Part model, mm, in its own coordinate system. Face numbers are marked on the shaded views. A direction names the side the tool comes from. Give positions to 0.01 mm unless a question says otherwise; leave off trailing zeros. Order: outer loops, then holes, each group sorted by start corner. A loop starts at its lowest first (then second) coordinate and runs counter-clockwise, first axis right, second up. Notation, with made-up numbers: (12.25, 4.25) -> (34.25, 4.25) arc R16 cw to (34.25, 30.25) -> close; hole circle Ø11 at (20, -1.5). An arc over 180 degrees is marked (long way). Write item = value, one per line. Start each with the question number.
Item 1: Band-saw the part on D-D on y = -137.5. Write the cut outline in (x, z), plus the area to 3 significant figures.
Item 2: Pull direction Z, two halves, no side cores. Call the marked faces 3, 4 and 5: +Z half, -Z half, draft (parallel to the pull), parting line (faces both ways), or undercut.
Item 3: Tool access for the marked faces 1 and 2: list every direction of +Z, -Z, +X, -X, +Y, -Y with a clear straight run to the whole face (end or side of a thin tool).
Item 4: Band-saw the part on A-A on y = -17.5. Write the cut outline in (x, z).
Item 5: Band-saw the part on B-B on z = 0. Write the cut outline in (x, y), plus the area to 3 significant figures.
Item 6: Band-saw the part on C-C on y = -70.5. Write the cut outline in (x, z).
Item 7: Flat gauge pins, fed straight in: P1, Ø18.5, axis at y = -13.5, z = -18, coming from the -X side; P2, Ø6, axis at x = 0, y = -126, coming from the -Z side; P3, Ø8, axis at x = 18, y = -43, coming from the +Z side. Where does each tip first touch, or does it go through?
Item 8: Drill centre lines: line 1 along X through (y, z) = (-29.5, 0); line 2 along Y through (x, z) = (0, 10). Where is each one in solid material? Low to high.
```python
from build123d import *

# Parameters (mm, degrees)
STOCKDIAMETER_R        = 22.5
BASESTOCK_DEPTH        = 150
DIAMETERCUT_START      = -25
SKETCH11_OUTSIDE_W     = 79.588
SKETCH11_OUTSIDE_H     = 79.588
SKETCH11_OUTSIDE_R     = 17.5
DIAMETERCUT_DEPTH      = 126
SHAFTHOLE_R            = 6
MOTOR1SHAFTHOLE_DEPTH  = 151
SKETCH10_W             = 4
SKETCH10_H             = 20
SHAFTKEY_DEPTH         = 23.5
SHAFTKEY_DEPTH_BACK    = 23.5
ARMKEY_START           = -150
ARMKEYSKETCH_W         = 60
ARMKEYSKETCH_H         = 20
ARMKEY_DEPTH           = 50
ARM1MOUNTINGHOLE_START = 15
SKETCH13_R             = 5
ARM1MOUNTINGHOLE_DEPTH = 11.683375
FILLET1_R              = 1


with BuildPart() as part:
    # StockDiameter → BaseStock (new body)
    with BuildSketch(Plane(origin=(0, 0, 0), x_dir=(1, 0, 0), z_dir=(0, 1, 0))):
        Circle(STOCKDIAMETER_R)
    extrude(amount=-BASESTOCK_DEPTH)

    # Sketch11 outside → DiameterCut (cut, through all)
    with BuildSketch(Plane(origin=(0, 0, 0), x_dir=(1, 0, 0), z_dir=(0, 1, 0)).offset(DIAMETERCUT_START)):
        Rectangle(SKETCH11_OUTSIDE_W, SKETCH11_OUTSIDE_H)
        Circle(SKETCH11_OUTSIDE_R, mode=Mode.SUBTRACT)
    extrude(amount=-DIAMETERCUT_DEPTH, mode=Mode.SUBTRACT)

    # ShaftHole → Motor1ShaftHole (cut, through all)
    with BuildSketch(Plane(origin=(0, 0, 0), x_dir=(1, 0, 0), z_dir=(0, 1, 0))):
        Circle(SHAFTHOLE_R)
    extrude(amount=-MOTOR1SHAFTHOLE_DEPTH, mode=Mode.SUBTRACT)

    # Sketch10 → ShaftKey (cut, two sides)
    with BuildSketch(Plane.XY) as shaftkey_sk:
        with Locations((0, -10)):
            Rectangle(SKETCH10_W, SKETCH10_H)
    extrude(amount=SHAFTKEY_DEPTH, mode=Mode.SUBTRACT)
    extrude(shaftkey_sk.sketch, amount=-SHAFTKEY_DEPTH_BACK, mode=Mode.SUBTRACT)

    # ArmKeySketch → ArmKey (cut)
    with BuildSketch(Plane(origin=(0, 0, 0), x_dir=(1, 0, 0), z_dir=(0, 1, 0)).offset(ARMKEY_START)):
        with Locations((0, -25)):
            Rectangle(ARMKEYSKETCH_W, ARMKEYSKETCH_H)
    extrude(amount=ARMKEY_DEPTH, mode=Mode.SUBTRACT)

    # Sketch13 → Arm1MountingHole (cut)
    with BuildSketch(Plane.XY.offset(ARM1MOUNTINGHOLE_START)):
        with Locations((0, -126)):
            Circle(SKETCH13_R)
    extrude(amount=-ARM1MOUNTINGHOLE_DEPTH, mode=Mode.SUBTRACT)

    # Fillet1
    fillet1_edges = [part.edges().sort_by_distance(p)[0] for p in [
        (-22.5, -25, 0),
    ]]
    fillet(fillet1_edges, radius=FILLET1_R)


solid = part.part
```
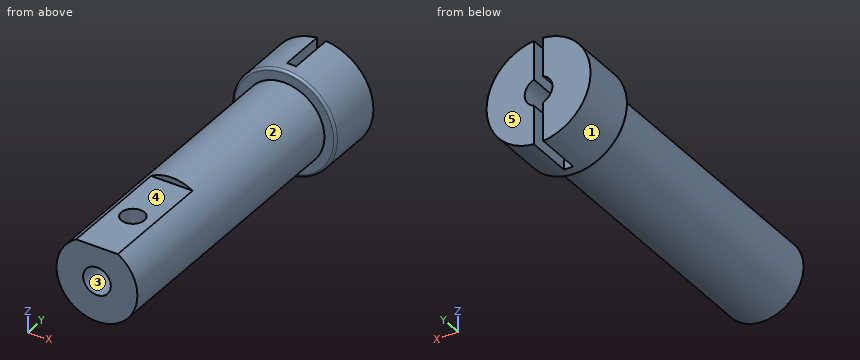
Values found:
q1.outline = (-9.01, 15) arc R17.5 ccw (long way) to (9.01, 15) -> close; hole circle Ø12 at (0, 0)
q1.area = 819 mm^2
q2.face_3 = undercut
q2.face_4 = +Z half
q2.face_5 = draft
q3.face_1 = +Y, -Y
q3.face_2 = -Y
q4.outline = (-2, -22.41) -> (-2, -5.66) arc R6 cw to (-2, 5.66) -> (-2, 22.41) arc R22.5 ccw to start; (2, -22.41) arc R22.5 ccw to (2, 22.41) -> (2, 5.66) arc R6 cw to (2, -5.66) -> close
q5.outline = (-22.5, -24) arc R1 ccw to (-21.5, -25) -> (-17.5, -25) -> (-17.5, -150) -> (-6, -150) -> (-6, 0) -> (-22.5, 0) -> close; (6, -150) -> (17.5, -150) -> (17.5, -25) -> (21.5, -25) arc R1 ccw to (22.5, -24) -> (22.5, 0) -> (6, 0) -> close
q5.area = 3,700 mm^2
q6.outline = circle Ø35 at (0, 0); hole circle Ø12 at (0, 0)
q7.P1 = -20.73
q7.P2 = -17.5
q7.P3 = 10.5
q8.line_1 = -17.5 to -6, 6 to 17.5
q8.line_2 = -150 to -131, -121 to -20
